Study the drawing (mm; zero at the part's minimum x, y, z) and answer. A direction names the side the tool comes from. Coordinates: 2 decimals unless noted, no trailing zeros. Write each loop counter-clockwise with the first axis right and the second up, starting at its lowest first coordinate (ties: lowest second). Pieces come first, ordered by that corner, then holes. Notation, with made-up numbers: (9.25, 31) -> (25.25, 31) arc R23 cw to (25.25, 44) -> close; hole circle Ø7 at (-35.5, 58). An arc over 180 degrees is marked (long way). Write item = value, one per line. Start each with the question number.
1) Section D-D (y = 26) is taken. Determine the outline of the cut face in (x, z), plus the area to 3 significant figures.
2) Section A-A (x = 2.99) is taken. Determine the outline of the cut face in (y, z), plus the area to 3 significant figures.
3) Find the intervals of material crossed by line 1 along X through (y, z) = (41.2, 10); line 2 along Z through (x, y) = (11.5, 40.55); line 3 along Y through (x, z) = (2.99, 2.1), in increasing order. Write a range as from..to.
4) Flat-ended cylindrical pins translate along their axes: pin 1 Ø3.5 at (x, y) = (2.99, 34.1) entering from -Z; pin 2 Ø8 at (x, y) = (13.5, 23.5) entering from -Z; pin 3 Ø7 at (x, y) = (13, 16.5) entering from +Z; pin 4 Ø3 at (y, z) = (28.5, 16) entering from -X. Find the tip coordinate at first contact, or state that the pin passes through.
5) A tool of negligible diameter and unlimited length cuts with its end or side. For the marked faces 1 and 2, from which of +Z, -Z, +X, -X, +Y, -Y can it reach the whole face along a straight path? Write none if from no direction.
6) Section B-B (z = 10) is taken. Determine the outline of the cut face in (x, y), plus the area to 3 significant figures.
7) Section C-C (x = 20.5) is taken. Determine the outline of the cut face in (y, z).
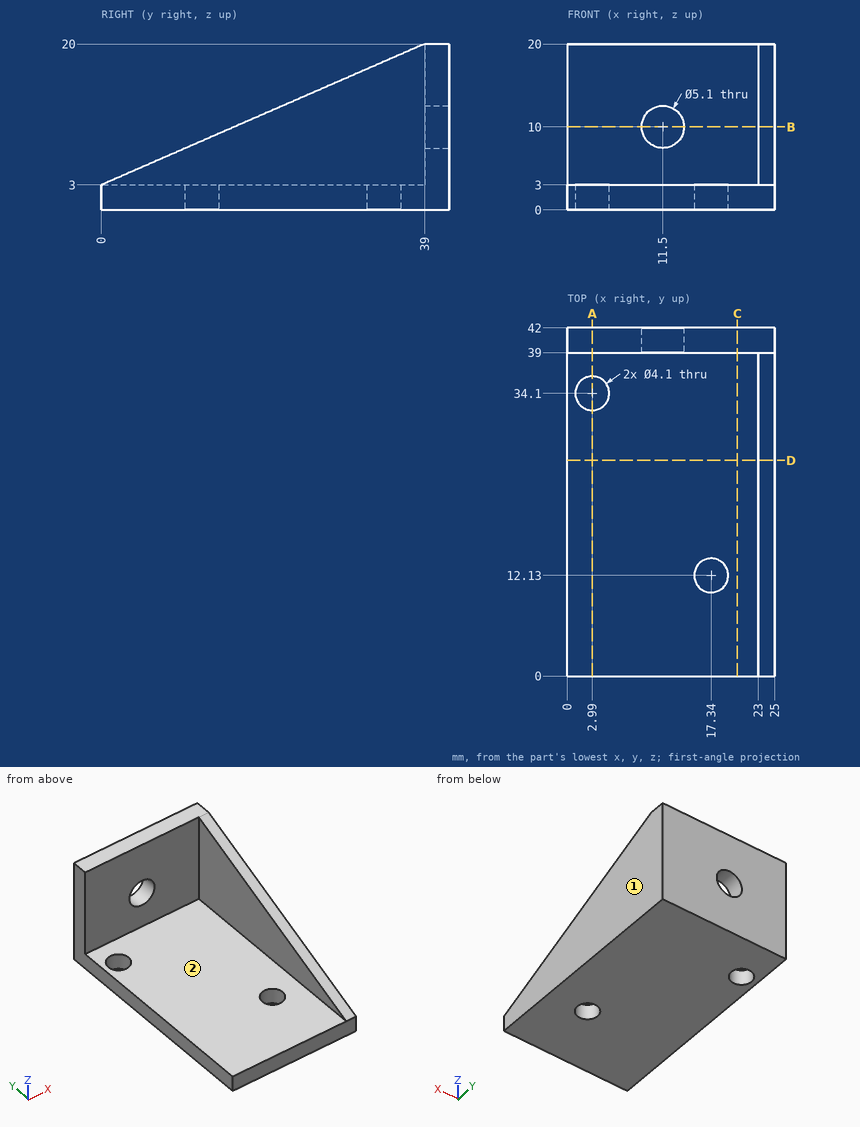
Answer key:
q1.outline = (0, 0) -> (25, 0) -> (25, 14.33) -> (23, 14.33) -> (23, 3) -> (0, 3) -> close
q1.area = 97.7 mm^2
q2.outline = (0, 0) -> (32.05, 0) -> (32.05, 3) -> (0, 3) -> close; (36.15, 0) -> (42, 0) -> (42, 20) -> (39, 20) -> (39, 3) -> (36.15, 3) -> close
q2.area = 165 mm^2
q3.line_1 = 0..8.95, 14.05..25
q3.line_2 = 0..7.45, 12.55..20
q3.line_3 = 0..32.05, 36.15..42
q4.pin_1 = through
q4.pin_2 = 0
q4.pin_3 = 3
q4.pin_4 = 23
q5.face_1 = +Z, -Z, +X, +Y, -Y
q5.face_2 = +Z, -X, -Y
q6.outline = (0, 39) -> (8.95, 39) -> (8.95, 42) -> (0, 42) -> close; (14.05, 39) -> (23, 39) -> (23, 16.06) -> (25, 16.06) -> (25, 42) -> (14.05, 42) -> close
q6.area = 106 mm^2
q7.outline = (0, 0) -> (42, 0) -> (42, 20) -> (39, 20) -> (39, 3) -> (0, 3) -> close
